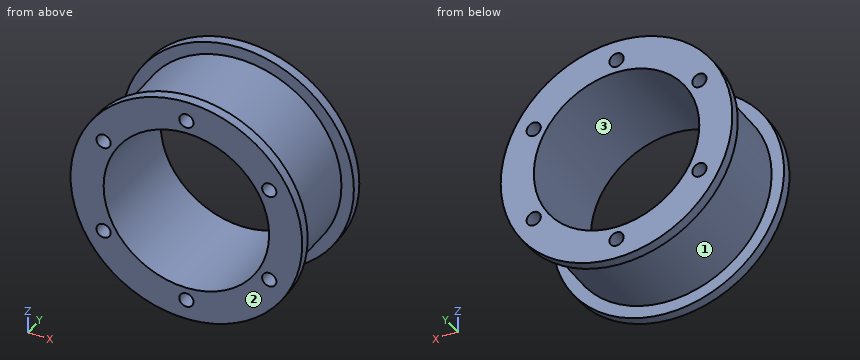
from build123d import *

# Parameters (mm, degrees)
F0_R     = 35.56
F0_R_2   = 25.4
F1_DEPTH = 3.175
F2_R     = 31.75
F2_R_2   = 25.4
F3_DEPTH = 26.9875
F4_R     = 35.56
F4_R_2   = 25.4
F5_DEPTH = 3.175
F6_R     = 2.18313
F7_DEPTH = 33.3385


with BuildPart() as f1:
    # F0 (on Front) → F1 (new body)
    with BuildSketch(Plane.XZ):
        Circle(F0_R)
        Circle(F0_R_2, mode=Mode.SUBTRACT)
    extrude(amount=F1_DEPTH)

    # F2 (on face) → F3 (join)
    with BuildSketch(Plane.XZ.offset(3.175)):
        Circle(F2_R)
        Circle(F2_R_2, mode=Mode.SUBTRACT)
    extrude(amount=F3_DEPTH)

    # F4 (on face) → F5 (join)
    with BuildSketch(Plane.XZ.offset(30.1625)):
        Circle(F4_R)
        Circle(F4_R_2, mode=Mode.SUBTRACT)
    extrude(amount=F5_DEPTH)

    # F6 (on face) → F7 (cut, through all)
    with BuildSketch(Plane.XZ.offset(33.3375)):
        with Locations((0, 29.36875)):
            Circle(F6_R)
        with Locations((-25.434084, 14.684375)):
            Circle(F6_R)
        with Locations((-25.434084, -14.684375)):
            Circle(F6_R)
        with Locations((0, -29.36875)):
            Circle(F6_R)
        with Locations((25.434084, -14.684375)):
            Circle(F6_R)
        with Locations((25.434084, 14.684375)):
            Circle(F6_R)
    extrude(amount=-F7_DEPTH, mode=Mode.SUBTRACT)


solid = f1.part
Part model, mm, in its own coordinate system. Face numbers are marked on the shaded views. Give positions to 0.01 mm unless a question says otherwise; leave off trailing zeros. Order: outer loops, then holes, each group sorted by start corner. A loop starts at its lowest first (then second) coordinate and runs counter-clockwise, first axis right, second up. Notation, with made-up numbers: (45.5, 20) - (56.5, 20) arc R19 cw to (56.5, 31) - close; hole circle Ø7 at (19.25, 34.25). An arc over 180 degrees is marked (long way). One line per question, with ' | ' between items.
1. Drill centre lines: probe 1 along Z at (x, y) = (0, -14); probe 2 along X at (y, z) = (-11, 15); probe 3 along Y at (x, z) = (-6, 33.5) (1 decimal). Where is each one in solid material? Low to high.
Filled in:
probe 1: -31.75 to -31.55, -27.19 to -25.4, 25.4 to 27.19, 31.55 to 31.75 | probe 2: -27.98 to -27.59, -23.27 to -20.5, 20.5 to 23.27, 27.59 to 27.98 | probe 3: -33.3 to -30.2, -3.2 to 0
2. Pull direction Z, two halves, no side cores. Call the marked faces 1, 2 and 3: +Z half, -Z half, draft (parallel to the pull), parting line (faces both ways), or undercut.
Filled in:
face 1: parting line | face 2: draft | face 3: undercut
3. Band-saw the part on C-C on x = 8.5. List the corners of the cut face in (y, z) (1 decimal), then the cut area to 3 significant figures.
Filled in:
outline: (-33.3, -34.5) - (-30.2, -34.5) - (-30.2, -30.6) - (-3.2, -30.6) - (-3.2, -34.5) - (0, -34.5) - (0, -23.9) - (-33.3, -23.9) - close; (-33.3, 23.9) - (0, 23.9) - (0, 34.5) - (-3.2, 34.5) - (-3.2, 30.6) - (-30.2, 30.6) - (-30.2, 34.5) - (-33.3, 34.5) - close | area: 494 mm²
4. Band-saw the part on A-A on x = 0. Give the number of separate pieces and of enclosed holes in the cut face, then the cut area to 3 significant figures.
Filled in:
separate pieces: 4 | enclosed holes: 0 | area: 181 mm²
5. Drop flat-ended pins along their axis: P1, Ø3.5, axis at x = 0, z = -29.37, coming from the +Y side; P2, Ø10, axis at y = -4, z = -22, coming from the -X side; P3, Ø4, axis at y = -4, z = 16.5, coming from the +X side; P4, Ø3, axis at x = 27.5, y = -29.5, coming from the +Z side. Give the stop position or say it passes through.
Filled in:
P1: through | P2: x = -31.2 | P3: x = 32.39 | P4: z = 24.09
6. Band-saw the part on D-D on y = -15. List the corners of the cut face in (x, z), then the cut area to 3 significant figures.
Filled in:
outline: circle Ø63.5 at (0, 0); hole circle Ø4.37 at (-25.43, -14.68); hole circle Ø4.37 at (-25.43, 14.68); hole circle Ø50.8 at (0, 0); hole circle Ø4.37 at (0, -29.37); hole circle Ø4.37 at (0, 29.37); hole circle Ø4.37 at (25.43, -14.68); hole circle Ø4.37 at (25.43, 14.68) | area: 1,050 mm²
